Can you work these out from the model? Positions are in its coordinate system, mm. Coordinates: 2 decimals unless noted, no trailing zeros. Loops run counter-clockwise (first coordinate to the right, second up) from the corner with the lowest first, then second, coordinate; pieces in that order, holes last.
```python
from build123d import *

# Parameters (mm, degrees)
SKETCH_2_R      = 1.5
SKETCH_2_R_2    = 1.6
EXTRUDE_2_DEPTH = 2
FILLET_1_R      = 1
FILLET_2_R      = 20


with BuildPart() as part:
    # 草图2 → 凸台-拉伸2 (new body)
    with BuildSketch(Plane(origin=(0, 0, 0), x_dir=(1, 0, 0), z_dir=(0, 1, 0))):
        with BuildLine():
            Line((20.5, 3), (-3, 3))
            Line((-3, 3), (-3, -3))
            Line((-3, -3), (20.5, -3))
            Line((20.5, -3), (48.853509418, -0.484348264))
            ThreePointArc((48.853509418, -0.484348264), (52.49608515, 3.676927871), (48.5, 7.5))
            Line((48.5, 7.5), (20.5, 7.5))
            Line((20.5, 7.5), (20.5, 3))
        make_face()
        with Locations(Location((0, 0, 0), (0, 0, 90))):
            Circle(SKETCH_2_R, mode=Mode.SUBTRACT)
        with Locations(Location((15, 0, 0), (0, 0, 90))):
            Circle(SKETCH_2_R, mode=Mode.SUBTRACT)
        with Locations(Location((48.5, 3.5, 0), (0, 0, 270))):
            Circle(SKETCH_2_R_2, mode=Mode.SUBTRACT)
    extrude(amount=EXTRUDE_2_DEPTH)

    # 圆角1
    fillet_1_edges = [part.edges().sort_by_distance(p)[0] for p in [
        (20.5, 1, -3),
    ]]
    fillet(fillet_1_edges, radius=FILLET_1_R)

    # 圆角2
    # the kernel refuses this fillet: 20 mm, written as the material it takes off along each edge
    with BuildSketch(Plane(origin=(20.5, -2.213765024, 3), x_dir=(0.9960870660689326, 0, -0.08837735462314833), z_dir=(0, 1, 0))) as fillet_2_piece_1:
        with BuildLine():
            CenterArc((FILLET_2_R * 0.0442753004743, FILLET_2_R), FILLET_2_R, 264.929735646, 5.070264354)
            Line((-FILLET_2_R * 0.0441020541488, FILLET_2_R * 0.00391293393107), (0, 0))
            Line((0, 0), (FILLET_2_R * 0.0442753004743, 0))
        make_face()
    extrude(amount=6.427530047, mode=Mode.SUBTRACT)


solid = part.part
```
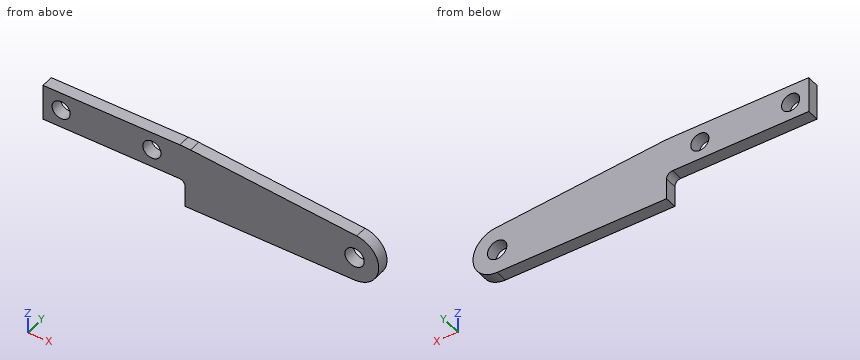
(1) I want a section at C-C on z = -3.5. Write out the boundary of the cut face in (x, y).
Check values:
outline: (20.37, 0) - (46.9, 0) - (46.9, 2) - (20.37, 2) - close; (50.1, 0) - (52.5, 0) - (52.5, 2) - (50.1, 2) - close
(2) I want a section at A-A on x = 15. Write out the boundary of the cut face in (y, z), then the cut area to 3 significant figures.
Check values:
outline: (0, -3) - (2, -3) - (2, -1.5) - (0, -1.5) - close; (0, 1.5) - (2, 1.5) - (2, 3) - (0, 3) - close
area: 6.00 mm2
(3) I want a section at B-B on y = 0.4. Write out the boundary of the cut face in (x, z).
Check values:
outline: (-3, -3) - (19.5, -3) arc R1 cw to (20.5, -4) - (20.5, -7.5) - (48.5, -7.5) arc R4 ccw to (48.85, 0.48) - (21.38, 2.92) arc R20 ccw to (19.61, 3) - (-3, 3) - close; hole circle Ø3 at (0, 0); hole circle Ø3 at (15, 0); hole circle Ø3.2 at (48.5, -3.5)
(4) If I drill on probe 1 along X at (y, z) = (1.25, 0); probe 2 along Z at (x, y) = (10.5, 0.9); probe 3 along X at (y, z) = (1, -4.5), over which ranges is the centre line in solid material (lowest first)?
Check values:
probe 1: x = -3 to -1.5, 1.5 to 13.5, 16.5 to 50.44
probe 2: z = -3 to 3
probe 3: x = 20.5 to 47.25, 49.75 to 52.37
(5) I want a section at D-D on z = 0. Write out the boundary of the cut face in (x, y), then the cut area to 3 significant figures.
Check values:
outline: (-3, 0) - (-1.5, 0) - (-1.5, 2) - (-3, 2) - close; (1.5, 0) - (13.5, 0) - (13.5, 2) - (1.5, 2) - close; (16.5, 0) - (50.44, 0) - (50.44, 2) - (16.5, 2) - close
area: 94.9 mm2
(6) I'm going to push flat-ended pins straight in: pin 1 (2.5 mm diameter, centred on x = 0, z = 0, fed in from -Y); pin 2 (0.6 mm diameter, centred on x = 10.5, y = 1, fed in from -Z). Where does each tip first touch, or does it pass through?
Check values:
pin 1: passes through
pin 2: stops at z = -3
